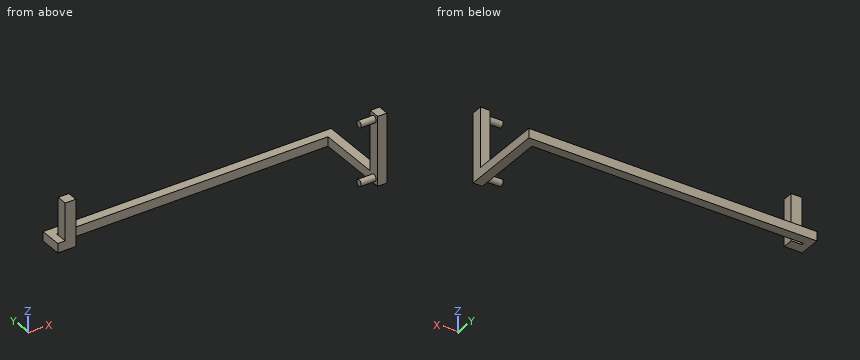
```python
from build123d import *

# Parameters (mm, degrees)
BOSS_EXTRUDE1_DEPTH = 5
SKETCH2_W           = 5.7
SKETCH2_H           = 5.7
BOSS_EXTRUDE2_DEPTH = 20
SKETCH3_W           = 5
SKETCH3_H           = 6
BOSS_EXTRUDE3_DEPTH = 32
SKETCH4_R           = 1.75
BOSS_EXTRUDE4_DEPTH = 8


with BuildPart() as part:
    # Sketch1 → Boss-Extrude1 (new body)
    with BuildSketch(Plane.XY):
        Polygon((0, 5.7), (0, 6.9), (5.5, 6.9), (145.5, 6.9), (145.5, -33.1), (150.5, -33.1), (150.5, 6.9), (150.5, 11.9), (5.5, 11.9), (-4, 11.9), (-4, 0), (0, 0), (5.7, 0), (5.7, 5.7), align=None)
    extrude(amount=BOSS_EXTRUDE1_DEPTH)

    # Sketch2 → Boss-Extrude2 (add)
    with BuildSketch(Plane.XY.offset(5)):
        with Locations((2.85, 2.85)):
            Rectangle(SKETCH2_W, SKETCH2_H)
    extrude(amount=BOSS_EXTRUDE2_DEPTH)

    # Sketch3 → Boss-Extrude3 (add)
    with BuildSketch(Plane.XY.offset(5)):
        with Locations((148, -30.1)):
            Rectangle(SKETCH3_W, SKETCH3_H)
    extrude(amount=BOSS_EXTRUDE3_DEPTH)

    # Sketch4 → Boss-Extrude4 (add)
    with BuildSketch(Plane.ZY.offset(-145.5)):
        with Locations(Location((3, -30.1, 0), (0, 0, 180))):
            Circle(SKETCH4_R)
        with Locations(Location((34, -30.1, 0), (0, 0, 180))):
            Circle(SKETCH4_R)
    extrude(amount=BOSS_EXTRUDE4_DEPTH)


solid = part.part
```
Geometry: final body of the model. Coordinates: model frame, mm. Round coordinates to 2 decimals unless told otherwise and drop trailing zeros. Write each loop counter-clockwise with the first axis right and the second up, starting at its lowest first coordinate (ties: lowest second). Pieces come first, ordered by that corner, then holes. Notation, with made-up numbers: M 56,84 L 75,84 A11 ccw 75,102 Z; hole C -40,-32 d6. An arc over 180 degrees is marked long. Answer in a Markdown table with one row per item. Add a question column.
(1) Cut plane D-D, the plane x = 74. Return the cut outline in (y, z), then the cut area to 3 significant figures.
(2) Contact query for flat-ended pins moving along their axis: pin 1 (1.7 mm diameter, centred on x = 2, z = 15, fed in from +Y); pin 2 (1.7 mm diameter, centred on y = 1.5, z = 16.5, fed in from +X); pin 3 (5 mm diameter, centred on x = 98.5, y = 6.5, fed in from +Z). Output: stop coordinate, or through.
(3) Cut plane A-A, the plane z = 23. Return the cut outline in (x, y), then the cut area to 3 significant figures.
(4) Cut plane C-C, the plane y = -30.1. Return the cut outline in (x, z).
(5) Cut plane B-B, the plane z = 3. Return the cut outline in (x, y), then the cut area to 3 significant figures.
(6) Ray query, L1, parallel to X at y = -29.5, z = 5; L2, parallel to X at y = -29, z = 34; L3, parallel to Y at x = 5.5, z = 10. Return the intervals inside material, ascending.
Established:
| question | item | result |
|---|---|---|
| 1 | outline | M 6.9,0 L 11.9,0 L 11.9,5 L 6.9,5 Z |
| 1 | area | 25.0 mm² |
| 2 | pin 1 | y = 5.7 |
| 2 | pin 2 | x = 5.7 |
| 2 | pin 3 | z = 5 |
| 3 | outline | M 0,0 L 5.7,0 L 5.7,5.7 L 0,5.7 Z; M 145.5,-33.1 L 150.5,-33.1 L 150.5,-27.1 L 145.5,-27.1 Z |
| 3 | area | 62.5 mm² |
| 4 | outline | M 137.5,1.25 L 145.5,1.25 L 145.5,0 L 150.5,0 L 150.5,37 L 145.5,37 L 145.5,35.75 L 137.5,35.75 L 137.5,32.25 L 145.5,32.25 L 145.5,4.75 L 137.5,4.75 Z |
| 5 | outline | M -4,0 L 5.7,0 L 5.7,5.7 L 0,5.7 L 0,6.9 L 145.5,6.9 L 145.5,-28.35 L 137.5,-28.35 L 137.5,-31.85 L 145.5,-31.85 L 145.5,-33.1 L 150.5,-33.1 L 150.5,11.9 L -4,11.9 Z |
| 5 | area | 1,060 mm² |
| 6 | L1 | 145.5 to 150.5 |
| 6 | L2 | 137.5 to 150.5 |
| 6 | L3 | 0 to 5.7 |
